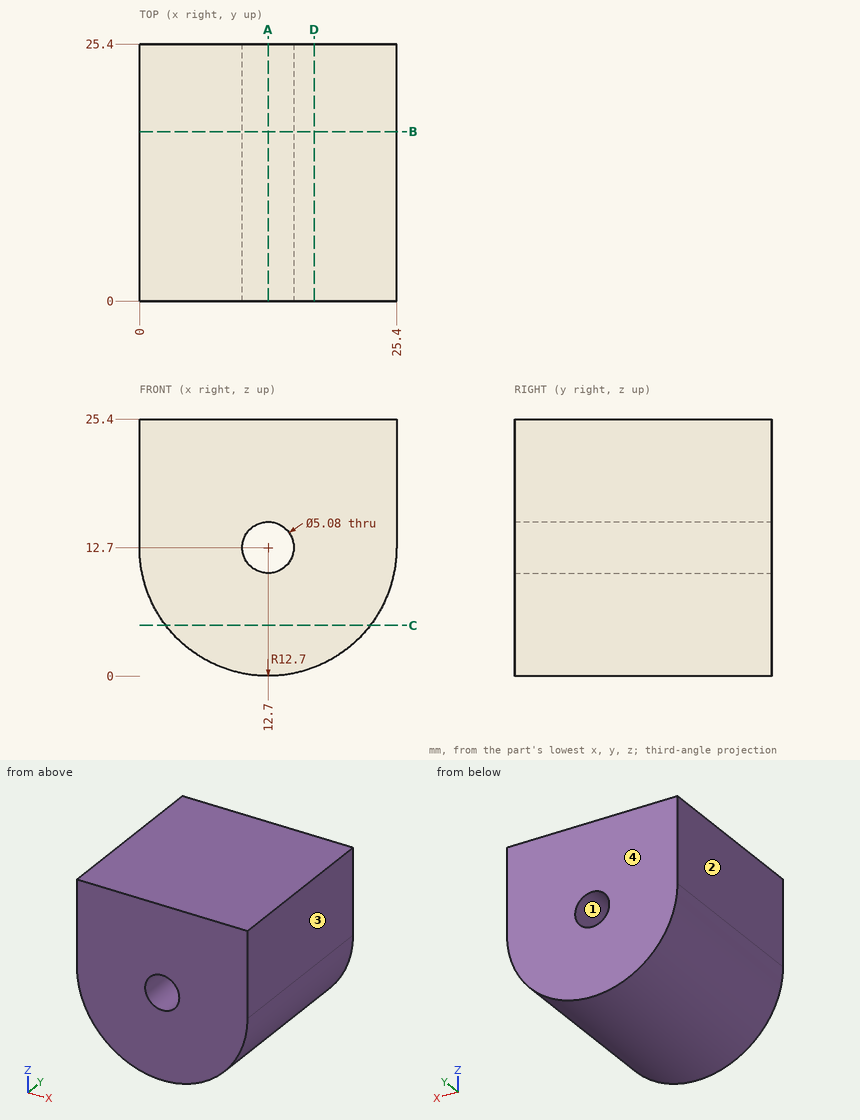
Could you check a few things on this drawing? It's one solid part, dimensions in mm from its lowest x, y, z. Give positions to 0.01 mm unless a question says otherwise; leave off trailing zeros. Order: outer loops, then holes, each group sorted by start corner. A loop starts at its lowest first (then second) coordinate and runs counter-clockwise, first axis right, second up. Notation, with made-up numbers: (-25, -5.5) - (9, -5.5) arc R16 cw to (9, -1.5) - close; hole circle Ø7 at (73.5, 11.25). An arc over 180 degrees is marked (long way). One line per item, written item: value. Start each with the question number.
1. If I drill on probe 1 along X at (y, z) = (14, 12.7); probe 2 along Z at (x, y) = (14.5, 14), over which ranges is the centre line in solid material (lowest first)?
2. For P1, Ø3, axis at x = 7.5, y = 18, coming from the -Z side, with a flat end and sliding along its axis, tell me the tip position at first contact or that it passes through.
3. Imagine slicing it at B-B on y = 16.75. List the corners of the cut face in (x, z) for me.
4. Thinking about a two-plate mould opening in X: for the marked faces 1, 2, 3 and 4, which applies, +X half, -X half, draft (parallel to the pull), parting line (faces both ways), or undercut?
5. Imagine slicing it at A-A on x = 12.7. List the corners of the cut face in (y, z) for me, plus the area to 3 significant figures.
6. Imagine slicing it at C-C on z = 5. List the corners of the cut face in (x, y) for me, plus the area to 3 significant figures.
7. Imagine slicing it at D-D on x = 17.25. List the corners of the cut face in (y, z) for me, plus the area to 3 significant figures.
Values:
1. probe 1: 0 to 10.16, 15.24 to 25.4
1. probe 2: 0.13 to 10.91, 14.49 to 25.4
2. P1: z = 0.55
3. outline: (0, 12.7) arc R12.7 ccw to (25.4, 12.7) - (25.4, 25.4) - (0, 25.4) - close; hole circle Ø5.08 at (12.7, 12.7)
4. face 1: undercut
4. face 2: -X half
4. face 3: +X half
4. face 4: draft
5. outline: (0, 0) - (25.4, 0) - (25.4, 10.16) - (0, 10.16) - close; (0, 15.24) - (25.4, 15.24) - (25.4, 25.4) - (0, 25.4) - close
5. area: 516 mm²
6. outline: (2.6, 0) - (22.8, 0) - (22.8, 25.4) - (2.6, 25.4) - close
6. area: 513 mm²
7. outline: (0, 0.84) - (25.4, 0.84) - (25.4, 25.4) - (0, 25.4) - close
7. area: 624 mm²
